from build123d import *

# Parameters (mm, degrees)
F1_DEPTH      = 80
F2_R          = 20
F3_DEPTH      = 80
F2_R_2        = 15
F4_DEPTH      = 50.001
F4_DEPTH_BACK = 80.001


with BuildPart() as f1:
    # F0 (on Front) → F1 (new body, symmetric)
    with BuildSketch(Plane.XZ):
        Polygon((0, 0), (-150, 0), (-150, -50), (50, -50), (50, 30), (140, 30), (140, 80), (0, 80), align=None)
    extrude(amount=F1_DEPTH, both=True)

    # F2 (on face) → F3 (join)
    with BuildSketch(Plane.XY):
        with BuildLine():
            Line((0, -45), (0, 45))
            Line((0, 45), (-30, 45))
            ThreePointArc((-30, 45), (-75, 0), (-30, -45))
            Line((-30, -45), (0, -45))
        make_face()
        with Locations((-30, 0)):
            Circle(F2_R, mode=Mode.SUBTRACT)
    extrude(amount=F3_DEPTH)

    # F2 (on face) → F4 (cut, two sides)
    with BuildSketch(Plane.XY) as f4_sk:
        with Locations((-110, 40)):
            Circle(F2_R_2)
        with Locations((-110, -40)):
            Circle(F2_R_2)
        with Locations((100, -40)):
            Circle(F2_R_2)
        with Locations((100, 40)):
            Circle(F2_R_2)
        with Locations((-30, 0)):
            Circle(F2_R)
    extrude(amount=-F4_DEPTH, mode=Mode.SUBTRACT)
    extrude(f4_sk.sketch, amount=F4_DEPTH_BACK, mode=Mode.SUBTRACT)


solid = f1.part
The model under review builds one solid part; all positions refer to its coordinate system, in mm. A direction names the side the tool comes from. Coordinates: 2 decimals unless noted, no trailing zeros. Write each loop counter-clockwise with the first axis right and the second up, starting at its lowest first coordinate (ties: lowest second). Pieces come first, ordered by that corner, then holes. Notation, with made-up numbers: (-6, -16.5) - (52, -16.5) arc R30 cw to (52, 20.5) - close; hole circle Ø9 at (-15.75, 10.5). An arc over 180 degrees is marked (long way). Answer as a JSON object with one key per item and string values. Group by question number.
1. Add section C-C (y = 40). Give the boundary of the cut face in (x, z), plus the area to 3 significant figures.
2. Add section D-D (z = 17). Give the boundary of the cut face in (x, y).
3. Add section B-B (x = -110). Give the boundary of the cut face in (y, z).
4. To check wall thickness, follow probe 1 along Y at (x, z) = (100, 53.5); probe 2 along Y at (x, z) = (-30, -38); probe 3 along Z at (x, y) = (-136, 67.5). State the ranges of each line that lie inside material, in increasing order.
5. Clearance check with flat-ended pins moving along their axes: pin 1 Ø9 at (x, z) = (-21.5, 47) entering from -Y; pin 2 Ø10 at (y, z) = (-44, 41.5) entering from -X; pin 3 Ø9 at (x, z) = (-12.5, 37.5) entering from +Y. State where each tip first meets the part, or that it passes through.
6. Machinability: for faces 4 (the face through (-15, -45, 39)), 5 (the face through (-91, -1, 0)), 6 (the face through (0, 62, 41)), 7 (the face through (94, -1, 30)), which of the approach directions +Z, -Z, +X, -X, +Y, -Y give a long, thin tool a straight path to every point of the face, cutting with its end or side? Answer none if there is none.
7. Add section A-A (z = 69). Give the boundary of the cut face in (x, y).
8. Mouldability with a two-part tool opening along Y and no side actions: class faces 1 (the face through (-111.953, -25.128, -24.65)), 2 (the face through (50, -1, -11)), 3 (the face through (-74.99, 0.99, 39.44)) as pulls with the +Y half, pulls with the -Y half, needs draft (parallel to the pull), parting line crosses it, or undercut.
Findings:
{
 "1": {"outline": "(-150, -50) - (-125, -50) - (-125, 0) - (-150, 0) - close; (-95, -50) - (50, -50) - (50, 30) - (85, 30) - (85, 80) - (-50.62, 80) - (-50.62, 0) - (-95, 0) - close; (115, 30) - (140, 30) - (140, 80) - (115, 80) - close", "area": "19,500 mm²"},
 "2": {"outline": "(-30, -45) - (0, -45) - (0, -80) - (50, -80) - (50, 80) - (0, 80) - (0, 45) - (-30, 45) arc R45 ccw to start; hole circle Ø40 at (-30, 0)"},
 "3": {"outline": "(-80, -50) - (-55, -50) - (-55, 0) - (-80, 0) - close; (-25, -50) - (25, -50) - (25, 0) - (-25, 0) - close; (55, -50) - (80, -50) - (80, 0) - (55, 0) - close"},
 "4": {"probe 1": "-80 to -55, -25 to 25, 55 to 80", "probe 2": "-80 to -20, 20 to 80", "probe 3": "-50 to 0"},
 "5": {"pin 1": "y = -45", "pin 2": "x = -52.45", "pin 3": "y = 45"},
 "6": {"face 4": "+Z, -X, -Y", "face 5": "+Z, -X", "face 6": "+Z, -X, +Y", "face 7": "-Z, +X, +Y, -Y"},
 "7": {"outline": "(-30, -45) - (0, -45) - (0, -80) - (140, -80) - (140, 80) - (0, 80) - (0, 45) - (-30, 45) arc R45 ccw to start; hole circle Ø40 at (-30, 0); hole circle Ø30 at (100, -40); hole circle Ø30 at (100, 40)"},
 "8": {"face 1": "undercut", "face 2": "needs draft", "face 3": "parting line crosses it"}
}
